Source: three-view drawing plus pictorial views. Frame: mm from the lowest corner of the part. Give positions to 0.01 mm unless a question says otherwise; leave off trailing zeros. Loops run counter-clockwise (first coordinate to the right, second up) from the corner with the lowest first, then second, coordinate; pieces in that order, holes last.
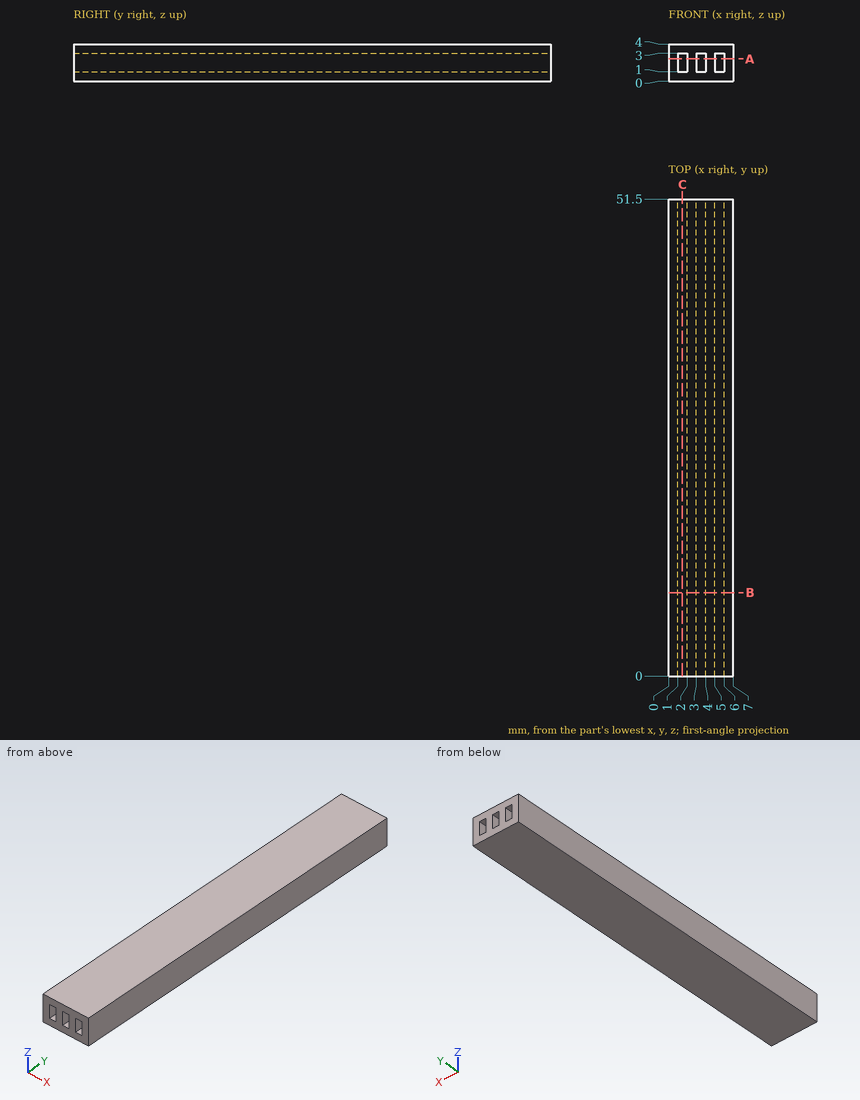
(1) Cut plane B-B (y = 9). Return the cut outline in (x, z), and give its area (3 significant figures).
Values follow:
outline: (0, 0) - (7, 0) - (7, 4) - (0, 4) - close; hole (1, 1) - (2, 1) - (2, 3) - (1, 3) - close; hole (3, 1) - (4, 1) - (4, 3) - (3, 3) - close; hole (5, 1) - (6, 1) - (6, 3) - (5, 3) - close
area: 22.0 mm2
(2) Ray query, probe 1 along X at (y, z) = (43, 2.6); probe 2 along Z at (x, y) = (5.25, 16). Return the intervals inside material, ascending.
Values follow:
probe 1: x = 0 to 1, 2 to 3, 4 to 5, 6 to 7
probe 2: z = 0 to 1, 3 to 4
(3) Pin query (flat end, axial travel): pin 1 Ø1 at (y, z) = (30, 0.5) entering from -X. Return the tip coordinate at first contact, or that it passes through.
Values follow:
pin 1: stops at x = 0
(4) Cut plane A-A (z = 2.4). Return the cut outline in (x, y), and give its area (3 significant figures).
Values follow:
outline: (0, 0) - (1, 0) - (1, 51.5) - (0, 51.5) - close; (2, 0) - (3, 0) - (3, 51.5) - (2, 51.5) - close; (4, 0) - (5, 0) - (5, 51.5) - (4, 51.5) - close; (6, 0) - (7, 0) - (7, 51.5) - (6, 51.5) - close
area: 206 mm2
(5) Cut plane C-C (x = 1.5). Return the cut outline in (y, z), and give its area (3 significant figures).
Values follow:
outline: (0, 0) - (51.5, 0) - (51.5, 1) - (0, 1) - close; (0, 3) - (51.5, 3) - (51.5, 4) - (0, 4) - close
area: 103 mm2
